For this review, take the finished solid that the model builds, in its own axes (mm). Face numbers are marked on the shaded views. A direction names the side the tool comes from. Give positions to 0.01 mm unless a question says otherwise; leave off trailing zeros. Order: outer loops, then holes, each group sorted by start corner. A loop starts at its lowest first (then second) coordinate and runs counter-clockwise, first axis right, second up. Notation, with made-up numbers: M -40,-13.5 L -14,-13.5 A16 ccw -14,-2.5 Z; hole C 58.25,37 d11. An arc over 180 degrees is marked long. Answer as CSV lines item,"result". Start each with the question number.
1. We need section C-C, the plane z = 4.75. Give the boundary of the cut face in (x, y) (3 decimals).
2. For line 1 along X through (y, z) = (-1, 6.5); line 2 along Y through (x, z) = (10.5, 2.75) (3 decimals), list the stretches that pass through material, from the lowest coordinate up.
3. We need section A-A, the plane y = 16.5. Give the boundary of the cut face in (x, z) (3 decimals).
4. Mouldability with a two-part tool opening along X and no side actions: class the marked faces 1, 2 and 3 as pulls with the +X half, pulls with the -X half, needs draft (parallel to the pull), parting line crosses it, or undercut.
5. Clearance check with a flat-ended pin moving along its axis: P1, Ø12, axis at x = -9.5, y = 12.5, coming from the -Z side. State where the tip first meets the part, or that it passes through.
6. Machinability: for the marked faces 4 and 5, which of the approach directions +Z, -Z, +X, -X, +Y, -Y give a long, thin tool a straight path to every point of the face, cutting with its end or side? Answer none if there is none.
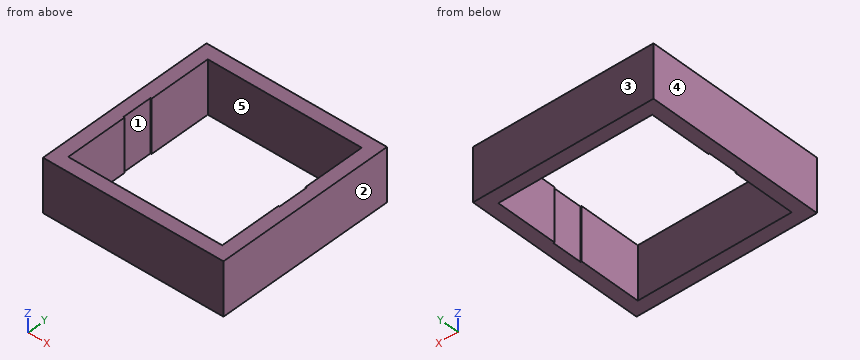
from build123d import *

# Parameters (mm, degrees)
F0_W     = 43.18
F0_H     = 43.18
F0_W_2   = 36.83
F0_H_2   = 36.83
F1_DEPTH = 12.7
F2_W     = 0.508
F2_H     = 7.112
F3_DEPTH = 12.701


with BuildPart() as f1:
    # F0 (on Top) → F1 (new body)
    with BuildSketch(Plane.XY):
        Rectangle(F0_W, F0_H)
        Rectangle(F0_W_2, F0_H_2, mode=Mode.SUBTRACT)
    extrude(amount=F1_DEPTH)

    # F2 (on face) → F3 (cut, through all)
    with BuildSketch(Plane(origin=(0, 0, 0), x_dir=(1, 0, 0), z_dir=(0, 0, -1))):
        with Locations((18.415, 0)):
            Rectangle(F2_W, F2_H)
        with Locations((-18.415, 0)):
            Rectangle(F2_W, F2_H)
    extrude(amount=-F3_DEPTH, mode=Mode.SUBTRACT)


solid = f1.part
Result set:
1,outline,"M -21.59,-21.59 L 21.59,-21.59 L 21.59,21.59 L -21.59,21.59 Z; hole M -18.669,-3.556 L -18.415,-3.556 L -18.415,-18.415 L 18.415,-18.415 L 18.415,-3.556 L 18.669,-3.556 L 18.669,3.556 L 18.415,3.556 L 18.415,18.415 L -18.415,18.415 L -18.415,3.556 L -18.669,3.556 Z"
2,line 1,"-21.59 to -18.67, 18.67 to 21.59"
2,line 2,"-21.59 to -18.415, 18.415 to 21.59"
3,outline,"M -21.59,0 L -18.415,0 L -18.415,12.7 L -21.59,12.7 Z; M 18.415,0 L 21.59,0 L 21.59,12.7 L 18.415,12.7 Z"
4,face 1,"undercut"
4,face 2,"pulls with the +X half"
4,face 3,"needs draft"
5,P1,"z = 0"
6,face 4,"+Z, -Z, -X, +Y, -Y"
6,face 5,"+Z, -Z"
